Geometry: final body of the model. Coordinates: model frame, mm. Round coordinates to 2 decimals unless told otherwise and drop trailing zeros. Loops run counter-clockwise (first coordinate to the right, second up) from the corner with the lowest first, then second, coordinate; pieces in that order, holes last. Notation, with made-up numbers: (-5, 44.25) - (2, 44.25) arc R15 ccw to (2, 72.25) - close; hole circle Ø3 at (68.5, 2). An arc over 180 degrees is marked (long way). Return JSON: item names as keys, results as strings. Group by question number.
1. First-contact query: pin 1 Ø12 at (x, z) = (56, -41) entering from +Y; pin 2 Ø1.5 at (x, y) = (16.5, 0.5) entering from +Z; pin 3 Ø1.5 at (x, y) = (3.5, 2) entering from +Z. Flat tips, straight axial feed; report the tip coordinate or a pass-through.
2. Section A-A on y = 1.9. Return loops of the section in (x, z).
3. Material intervals for probe 1 along Z at (x, y) = (53, 0.35); probe 2 along X at (y, z) = (0.5, -21.5); probe 3 along Z at (x, y) = (7.5, 2.3), sorted ascending.
4. Section C-C on z = 9.5. Return loops of the section in (x, y).
5. Section D-D on x = 14. Return loops of the section in (y, z).
6. Section B-B on x = 59. Return loops of the section in (y, z), and give its area (3 significant figures).
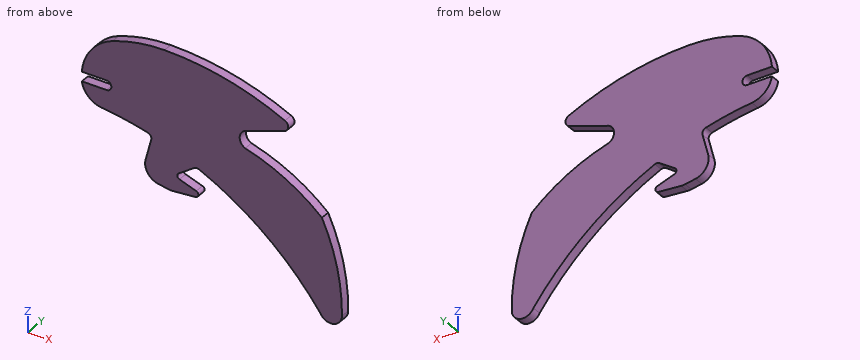
from build123d import *

# Parameters (mm, degrees)
BOSS_EXTRUDE1_DEPTH = 3
FILLET1_R           = 5
FILLET2_R           = 1
FILLET3_R           = 1.5


with BuildPart() as part:
    # Sketch1 → Boss-Extrude1 (new body)
    with BuildSketch(Plane(origin=(0, 0, 0), x_dir=(1, 0, 0), z_dir=(0, 1, 0))):
        with BuildLine():
            Line((0, 0), (7.87, 0))
            ThreePointArc((7.87, 0), (9.37, 1.5), (7.87, 3))
            Line((7.87, 3), (0, 3))
            ThreePointArc((0, 3), (2.150197581, 7.11318488), (6.36, 9.067463032))
            ThreePointArc((6.36, 9.067463032), (14.423757749, 10.275919643), (22.36, 12.146912791))
            Line((22.36, 12.146912791), (18.83, 25.66))
            Line((18.83, 25.66), (28.106454985, 27.26))
            Line((28.106454985, 27.26), (40.743591673, 26.19))
            Line((40.743591673, 26.19), (29.01, 22.19))
            Line((29.01, 22.19), (36.3, 17.207480276))
            ThreePointArc((36.3, 17.207480276), (57.98254967, 30.597458725), (75.506260733, 49.1))
            ThreePointArc((75.506260733, 49.1), (79.528190594, 51.04), (82.336251949, 47.568068084))
            ThreePointArc((82.336251949, 47.568068084), (80.805010077, 32.984321852), (76, 19.13))
            ThreePointArc((76, 19.13), (64.626879168, 11.098692866), (51.706470787, 5.910936222))
            ThreePointArc((51.706470787, 5.910936222), (49.97, 3.19), (51.706470787, 0.469063778))
            Line((51.706470787, 0.469063778), (64.104871289, -3.720532265))
            ThreePointArc((64.104871289, -3.720532265), (65.332594701, -5.328564668), (64.303533653, -7.070433303))
            ThreePointArc((64.303533653, -7.070433303), (45.731782679, -13.536259881), (26.199767539, -15.820385992))
            ThreePointArc((26.199767539, -15.820385992), (17.868444589, -15.127380639), (9.796210687, -12.952469527))
            ThreePointArc((9.796210687, -12.952469527), (3.000778454, -7.91122088), (0, 0))
        make_face()
    extrude(amount=BOSS_EXTRUDE1_DEPTH)

    # Fillet1
    fillet1_edges = [part.edges().sort_by_distance(p)[0] for p in [
        (18.83, 1.5, -25.66),
        (28.106454985, 1.5, -27.26),
    ]]
    fillet(fillet1_edges, radius=FILLET1_R)

    # Fillet2
    fillet2_edges = [part.edges().sort_by_distance(p)[0] for p in [
        (40.743591673, 1.5, -26.19),
        (29.01, 1.5, -22.19),
    ]]
    fillet(fillet2_edges, radius=FILLET2_R)

    # Fillet3
    fillet3_edges = [part.edges().sort_by_distance(p)[0] for p in [
        (22.36, 1.5, -12.146912791),
        (36.3, 1.5, -17.207480276),
    ]]
    fillet(fillet3_edges, radius=FILLET3_R)


solid = part.part
Taken from the geometry:
{
 "1": {"pin 1": "through", "pin 2": "z = 15.01", "pin 3": "z = 9.36"},
 "2": {"outline": "(0, -3) arc R7.22 ccw to (6.36, -9.07) arc R98.54 cw to (20.92, -11.75) arc R1.5 cw to (21.98, -13.58) - (20.21, -20.39) arc R5 ccw to (24.19, -26.59) - (27.47, -27.15) arc R5 ccw to (28.75, -27.21) - (35.99, -26.59) arc R1 ccw to (36.23, -24.65) - (30.9, -22.83) arc R1 cw to (30.66, -21.06) - (35.6, -17.69) arc R1.5 cw to (37.08, -17.56) arc R98.54 cw to (75.51, -49.1) arc R3.6 ccw to (82.34, -47.57) arc R64.11 ccw to (76, -19.13) arc R59.88 ccw to (51.71, -5.91) arc R3 cw to (51.71, -0.47) - (64.1, 3.72) arc R1.81 ccw to (64.3, 7.07) arc R90.13 ccw to (26.2, 15.82) arc R46.46 ccw to (9.8, 12.95) arc R15.05 ccw to (0, 0) - (7.87, 0) arc R1.5 cw to (7.87, -3) - close"},
 "3": {"probe 1": "-26.8 to -6.28, -0.03 to 11.54", "probe 2": "20.05 to 30.3, 44.72 to 77.08", "probe 3": "-9.2 to -3, 0 to 11.88"},
 "4": {"outline": "(4.39, 0) - (58.72, 0) - (58.72, 3) - (4.39, 3) - close"},
 "5": {"outline": "(0, -10.2) - (3, -10.2) - (3, 14.28) - (0, 14.28) - close"},
 "6": {"outline": "(0, -31.44) - (3, -31.44) - (3, -8.41) - (0, -8.41) - close; (0, 2) - (3, 2) - (3, 9.39) - (0, 9.39) - close", "area": "91.3 mm2"}
}
